```python
from build123d import *

# Parameters (mm, degrees)
SKETCH1_R           = 12.8
BOSS_EXTRUDE1_DEPTH = 3.18
CUT_EXTRUDE1_DEPTH  = 19.379129468
CIRPATTERN1_COUNT   = 30
SKETCH4_R           = 2.25
CUT_EXTRUDE3_DEPTH  = 19.349437359
BOSS_EXTRUDE6_START = -3.18
BOSS_EXTRUDE6_DEPTH = 3.18
SKETCH8_R           = 1.47
CUT_EXTRUDE4_DEPTH  = 54.506204937
SKETCH9_R           = 1.47
CUT_EXTRUDE5_DEPTH  = 54.506204937


with BuildPart() as part:
    # Sketch1 → Boss-Extrude1 (new body)
    with BuildSketch(Plane.XY):
        with Locations(Location((0, 0, 0), (0, 0, 180))):
            Circle(SKETCH1_R)
    extrude(amount=BOSS_EXTRUDE1_DEPTH)

    # Sketch2 → Cut-Extrude1 (cut, through all)
    with BuildSketch(Plane.XY.offset(3.18)):
        with BuildLine():
            ThreePointArc((-0.321034752, 10.995314306), (0, 11), (0.321034752, 10.995314306))
            ThreePointArc((0.321034752, 10.995314306), (0.594388904, 11.912556329), (1.044293354, 12.75732932))
            ThreePointArc((1.044293354, 12.75732932), (0, 12.8), (-1.044293354, 12.75732932))
            ThreePointArc((-1.044293354, 12.75732932), (-0.594388904, 11.912556329), (-0.321034752, 10.995314306))
        make_face()
    cut_extrude1 = extrude(amount=-CUT_EXTRUDE1_DEPTH, mode=Mode.SUBTRACT)

    # CirPattern1: Cut-Extrude1 ×30 about axis
    cirpattern1_axis = Axis((0, 0, 0), (0, 0, 1))
    for i in range(1, CIRPATTERN1_COUNT):
        add(cut_extrude1.rotate(cirpattern1_axis, i * 360 / CIRPATTERN1_COUNT), mode=Mode.SUBTRACT)

    # Sketch4 → Cut-Extrude3 (cut, through all)
    with BuildSketch(Plane.XY.offset(3.18)):
        Circle(SKETCH4_R)
    extrude(amount=-CUT_EXTRUDE3_DEPTH, mode=Mode.SUBTRACT)

    # Sketch6 → Boss-Extrude6 (add)
    with BuildSketch(Plane(origin=(0, 0, 0), x_dir=(-1, 0, 0), z_dir=(0, 0, -1)).offset(BOSS_EXTRUDE6_START)):
        with BuildLine():
            Line((-35.536396094, 30.96349829), (-0.895379942, 10.96349829))
            ThreePointArc((-0.895379942, 10.96349829), (-9.010672487, 6.3093408), (-10.608556418, -2.908355332))
            Line((-10.608556418, -2.908355332), (-41.250334142, 22.803149056))
            ThreePointArc((-41.250334142, 22.803149056), (-42.132156315, 29.501253453), (-35.536396094, 30.96349829))
        make_face()
    extrude(amount=BOSS_EXTRUDE6_DEPTH)

    # Sketch8 → Cut-Extrude4 (cut, through all)
    with BuildSketch(Plane.XY.offset(3.18)):
        with Locations((-3.173453683, 4.526502263)):
            Circle(SKETCH8_R)
        with Locations((3.173453683, -4.526502263)):
            Circle(SKETCH8_R)
    extrude(amount=-CUT_EXTRUDE4_DEPTH, mode=Mode.SUBTRACT)

    # Sketch9 → Cut-Extrude5 (cut, through all)
    with BuildSketch(Plane(origin=(0, 0, 0), x_dir=(-1, 0, 0), z_dir=(0, 0, -1))):
        with Locations((-38.393365118, 26.883323673)):
            Circle(SKETCH9_R)
    extrude(amount=-CUT_EXTRUDE5_DEPTH, mode=Mode.SUBTRACT)


solid = part.part
```
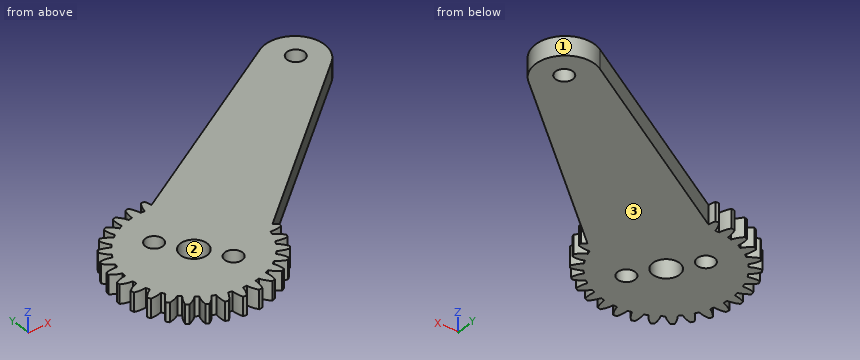
Build history of the part. All positions in model axes, mm. Face numbers are marked on the shaded views. Round coordinates to 2 decimals unless told otherwise and drop trailing zeros. Write each loop counter-clockwise with the first axis right and the second up, starting at its lowest first coordinate (ties: lowest second). Pieces come first, ordered by that corner, then holes.
1) Pin check, flat tip, straight feed: pin 1 (1.5 mm diameter, centred on x = -4.5, z = 0.5, fed in from -Y). Stop position of the tip, or through.
2) Band-saw the part on A-A, the plane y = 20. List the corners of the cut face in (x, z), and give its area (3 significant figures).
3) Band-saw the part on C-C, the plane x = 18. List the corners of the cut face in (y, z), and give its area (3 significant figures).
4) Mould opens along X. For the marked faces 1, 2 and 3 say: +X half, -X half, draft (parallel to the pull), parting line (faces both ways), or undercut.
5) Drill centre lines: probe 1 along Y at (x, z) = (-9.5, 2.1); probe 2 along Y at (x, z) = (-10, 0.35); probe 3 along Y at (x, z) = (0, 2.85). Where is each one in solid material? Low to high.
6) Band-saw the part on B-B, the plane z = 2.3. Give the number of separate pieces and of enclosed holes in the cut face, and give its area (3 significant figures).
Ans:
1. pin 1: stops at y = -12.24
2. outline: (16.55, 0) - (37.91, 0) - (37.91, 3.18) - (16.55, 3.18) - close
2. area: 67.9 mm2
3. outline: (3.29, 0) - (20.84, 0) - (20.84, 3.18) - (3.29, 3.18) - close
3. area: 55.8 mm2
4. face 1: parting line
4. face 2: undercut
4. face 3: draft
5. probe 1: y = -7.61 to -5.9, -5.55 to 5.55, 5.9 to 7.61
5. probe 2: y = -7.73 to -6.45, -5.32 to 5.32, 6.45 to 7.73
5. probe 3: y = -11 to -2.25, 2.25 to 11
6. separate pieces: 1
6. enclosed holes: 4
6. area: 919 mm2
